```python
from build123d import *

# Parameters (mm, degrees)
F0_W     = 44
F0_H     = 37
F1_DEPTH = 15.5
F2_SIZE2 = 8.5
F2_SIZE  = 12
F3_SIZE2 = 8.5
F3_SIZE  = 2
F4_W     = 36
F4_H     = 19
F5_DEPTH = 25
F6_R     = 4
F7_SIZE  = 1


with BuildPart() as f1:
    # F0 (on Top) → F1 (new body)
    with BuildSketch(Plane.XY):
        Rectangle(F0_W, F0_H)
    extrude(amount=F1_DEPTH)

    # F2
    f2_edges = [f1.edges().sort_by_distance(p)[0] for p in [
        (0, -18.5, 15.5),
    ]]
    f2_side = f1.faces().sort_by_distance((0, 0, 15.5))[0]
    chamfer(f2_edges, length=F2_SIZE, length2=F2_SIZE2, reference=f2_side)

    # F3
    f3_edges = [f1.edges().sort_by_distance(p)[0] for p in [
        (-22, 6, 15.5),
        (22, 6, 15.5),
        (0, 18.5, 15.5),
    ]]
    f3_side = f1.faces().sort_by_distance((0, 6, 15.5))[0]
    chamfer(f3_edges, length=F3_SIZE, length2=F3_SIZE2, reference=f3_side)

    # F4 (on face) → F5 (join)
    with BuildSketch(Plane.XY.offset(15.5)):
        with Locations((0, 5)):
            Rectangle(F4_W, F4_H)
    extrude(amount=F5_DEPTH)

    # F6
    f6_edges = [f1.edges().sort_by_distance(p)[0] for p in [
        (-18, -4.5, 28),
        (-18, 14.5, 28),
        (18, -4.5, 28),
        (18, 14.5, 28),
    ]]
    fillet(f6_edges, radius=F6_R)

    # F7
    f7_edges = [f1.edges().sort_by_distance(p)[0] for p in [
        (-22, 0, 0),
        (0, 18.5, 0),
        (22, 0, 0),
        (0, -18.5, 0),
    ]]
    chamfer(f7_edges, length=F7_SIZE)


solid = f1.part
```
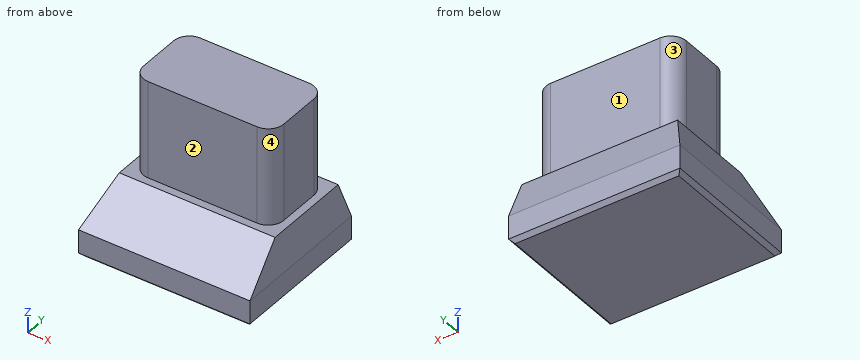
CAD build for the part. Positions are in the model's coordinates, mm. Face numbers are marked on the shaded views. A direction names the side the tool comes from. Give positions to 0.01 mm unless a question says otherwise; leave off trailing zeros. Order: outer loops, then holes, each group sorted by start corner. A loop starts at its lowest first (then second) coordinate and runs counter-clockwise, first axis right, second up.
(1) Saw through at A-A, the plane z = 28. Give the cut face in (x, y), then the cut area to 3 significant figures.
(2) Drill centre lines: L1, parallel to X at y = 5.5, z = 30.5; L2, parallel to Y at x = -8, z = 19.5; L3, parallel to Y at x = 3, z = 14.5. Where is each one in solid material? Low to high.
(3) Tool access for the marked faces 1, 2, 3 and 4: list every direction of +Z, -Z, +X, -X, +Y, -Y with a clear straight run to the whole face (end or side of a thin tool).
(4) Flat gauge pins, fed straight in: pin 1 (9 mm diameter, centred on y = 7.5, z = 32, fed in from -X); pin 2 (5.5 mm diameter, centred on y = 5, z = 22, fed in from +X); pin 3 (5 mm diameter, centred on x = 1.5, z = 21.5, fed in from -Y). Where does each tip first touch, or does it go through?
(5) Saw through at C-C, the plane x = -9. Give the cut face in (y, z), then the cut area to 3 significant figures.
(6) Saw through at B-B, the plane y = 2.5. Give the cut face in (x, z), then the cut area to 3 significant figures.
Results found:
1. outline: (-18, -0.5) arc R4 ccw to (-14, -4.5) - (14, -4.5) arc R4 ccw to (18, -0.5) - (18, 10.5) arc R4 ccw to (14, 14.5) - (-14, 14.5) arc R4 ccw to (-18, 10.5) - close
1. area: 670 mm2
2. L1: x = -18 to 18
2. L2: y = -4.5 to 14.5
2. L3: y = -7.91 to 16.74
3. face 1: +Z, +X, -X, +Y
3. face 2: +Z, +X, -X, -Y
3. face 3: +Z, -X, +Y
3. face 4: +Z, +X, -Y
4. pin 1: stops at x = -18
4. pin 2: stops at x = 18
4. pin 3: stops at y = -4.5
5. outline: (-18.5, 1) - (-17.5, 0) - (17.5, 0) - (18.5, 1) - (18.5, 7) - (16.5, 15.5) - (14.5, 15.5) - (14.5, 40.5) - (-4.5, 40.5) - (-4.5, 15.5) - (-6.5, 15.5) - (-18.5, 7) - close
5. area: 988 mm2
6. outline: (-22, 1) - (-21, 0) - (21, 0) - (22, 1) - (22, 7) - (20, 15.5) - (18, 15.5) - (18, 40.5) - (-18, 40.5) - (-18, 15.5) - (-20, 15.5) - (-22, 7) - close
6. area: 1,560 mm2
